Check sheet for the modelled part. Datum: model origin and axes. Units: mm. A direction names the side the tool comes from. Round coordinates to 2 decimals unless told otherwise and drop trailing zeros. Order: outer loops, then holes, each group sorted by start corner. A loop starts at its lowest first (then second) coordinate and runs counter-clockwise, first axis right, second up.
Q1. Set-up check for faces 4 (the flat face through (-301, 51, 18)), 5 (the cylindrical face through (-154, 53, 42)), 6 (the flat face through (-301, 51, -1)), 7 (the flat face through (-1, 51, 18)): record each of +Z, -Z, +X, -X, +Y, -Y from which the full face is reachable in a straight line by a thin tool's end or side.
Q2. Scan lines: probe 1 along Z at (x, y) = (-7, 50); probe 2 along Z at (x, y) = (-63.5, 12); probe 3 along X at (y, z) = (46, -14). Record each from-to range of solid material in increasing order.
Q3. Mould release check, pull along X, two halves, no side actions. Record for faces 1 (the flat face through (-152, 51, 0)), 2 (the flat face through (1, 50, -3)), 3 (the flat face through (-1, 40, -3)): +X half, -X half, draft (parallel to the pull), parting line (faces both ways), or undercut.
Q4. Depth check by flat-ended pin: P1, Ø7.5, axis at x = -261.47, y = 50, coming from the +Z side; P2, Ø5.5, axis at x = -38.53, y = 50, coming from the +Z side; P3, Ø8.5, axis at x = 38.53, y = 50, coming from the -Z side; P4, Ø4, axis at x = -305, y = 12.5, coming from the -Z side. Enter the tip coordinate at first touch or a pass-through.
Q5. Cross-section at C-C on y = 63.5. Record the cut outline in (x, z), then the cut area to 3 significant figures.
Q6. Cross-section at B-B on x = -150. Record the cut outline in (y, z).
Q7. Cross-section at A-A on z = -15. Record the cut outline in (x, y) (3 decimals).
Q8. Cross-section at D-D on z = 60. Record the cut outline in (x, y).
from build123d import *

# Parameters (mm, degrees)
SKETCH_1_R                         = 50
EXTRUDE_18_DEPTH                   = 13
EXTRUDE_18_2_DEPTH                 = 13
SKETCH_1_28_W                      = 300
SKETCH_1_28_H                      = 100
EXTRUDE_21_DEPTH                   = 15
SKETCH_1_30_R                      = 5
EXTRUDE_22_DEPTH                   = 70
SKETCH_1_31_R                      = 50
CUT_EXTRUDE_2_DEPTH                = 41
SKETCH_1_32_R                      = 50
EXTRUDE_23_DEPTH                   = 18
EXTRUDE_23_DEPTH_BACK              = 1
SKETCH_1_35_R                      = 3.175
CUT_EXTRUDE_5_DEPTH                = 130
CUT_EXTRUDE_5_DEPTH_BACK           = 69
SKETCH_1_36_R                      = 50
CUT_EXTRUDE_6_DEPTH                = 34
SKETCH_1_37_R                      = 50
EXTRUDE_24_DEPTH                   = 18
EXTRUDE_24_DEPTH_BACK              = 3
SKETCH_1_41_R                      = 3.175
CUT_EXTRUDE_7_DEPTH                = 87
CUT_EXTRUDE_7_DEPTH_BACK           = 98
THE_EXTENDED_SHAFT_CONNECTER_DEPTH = 36
SKETCH_3_R                         = 1.0922
CUT_EXTRUDE_8_DEPTH                = 31
SKETCH_5_R                         = 1.0922
SCREW_HOLES2_DEPTH                 = 47.995932


with BuildPart() as part:
    # Sketch 1 → Extrude 18 (new body)
    with BuildSketch(Plane.XY):
        with Locations((0, 50)):
            Circle(SKETCH_1_R)
    extrude(amount=EXTRUDE_18_DEPTH)



with BuildPart() as body_2:
    # Sketch 1 → Extrude 18 2 (new body)
    with BuildSketch(Plane.XY):
        with Locations((-300, 50)):
            Circle(SKETCH_1_R)
    extrude(amount=EXTRUDE_18_2_DEPTH)


with BuildPart() as part_1:
    add(part.part)

    add(body_2.part)  # Extrude 21 merges body 2
    # Sketch 1_28 → Extrude 21 (add)
    with BuildSketch(Plane.XY):
        with Locations((-150, 50)):
            Rectangle(SKETCH_1_28_W, SKETCH_1_28_H)
    extrude(amount=EXTRUDE_21_DEPTH)

    # Sketch 1_30 → Extrude 22 (add)
    with BuildSketch(Plane.XY):
        with Locations((-150, 50)):
            Circle(SKETCH_1_30_R)
    extrude(amount=EXTRUDE_22_DEPTH)

    # Sketch 1_31 → Cut-Extrude 2 (cut)
    with BuildSketch(Plane.XY):
        with Locations((-300, 50)):
            Circle(SKETCH_1_31_R)
    extrude(amount=CUT_EXTRUDE_2_DEPTH, mode=Mode.SUBTRACT)

    # Sketch 1_32 → Extrude 23 (add, two sides)
    with BuildSketch(Plane.XY) as extrude_23_sk:
        with Locations((-300, 50)):
            Circle(SKETCH_1_32_R)
    extrude(amount=EXTRUDE_23_DEPTH)
    extrude(extrude_23_sk.sketch, amount=-EXTRUDE_23_DEPTH_BACK)

    # Sketch 1_35 → Cut-Extrude 5 (cut, two sides)
    with BuildSketch(Plane.XY) as cut_extrude_5_sk:
        with Locations((-261.469660941, 50)):
            Circle(SKETCH_1_35_R)
    extrude(amount=CUT_EXTRUDE_5_DEPTH, mode=Mode.SUBTRACT)
    extrude(cut_extrude_5_sk.sketch, amount=-CUT_EXTRUDE_5_DEPTH_BACK, mode=Mode.SUBTRACT)

    # Sketch 1_36 → Cut-Extrude 6 (cut)
    with BuildSketch(Plane.XY):
        with Locations((0, 50)):
            Circle(SKETCH_1_36_R)
    extrude(amount=CUT_EXTRUDE_6_DEPTH, mode=Mode.SUBTRACT)

    # Sketch 1_37 → Extrude 24 (add, two sides)
    with BuildSketch(Plane.XY) as extrude_24_sk:
        with Locations((0, 50)):
            Circle(SKETCH_1_37_R)
    extrude(amount=EXTRUDE_24_DEPTH)
    extrude(extrude_24_sk.sketch, amount=-EXTRUDE_24_DEPTH_BACK)

    # Sketch 1_41 → Cut-Extrude 7 (cut, two sides)
    with BuildSketch(Plane.XY) as cut_extrude_7_sk:
        with Locations((-272.75493597, 77.24506403)):
            Circle(SKETCH_1_41_R)
        with BuildLine():
            ThreePointArc((-296.825, 88.530339059), (-297.75493597, 90.77540309), (-300, 91.705339059))
            Line((-300, 91.705339059), (-300, 85.355339059))
            ThreePointArc((-300, 85.355339059), (-297.75493597, 86.285275029), (-296.825, 88.530339059))
        make_face()
        with BuildLine():
            Line((-300, 85.355339059), (-300, 91.705339059))
            ThreePointArc((-300, 91.705339059), (-303.175, 88.530339059), (-300, 85.355339059))
        make_face()
        with Locations((-327.24506403, 77.24506403)):
            Circle(SKETCH_1_41_R)
        with Locations((-338.530339059, 50)):
            Circle(SKETCH_1_41_R)
        with BuildLine():
            ThreePointArc((-325, 25), (-329.490128061, 25), (-329.490128061, 20.509871939))
            Line((-329.490128061, 20.509871939), (-325, 25))
        make_face()
        with BuildLine():
            Line((-325, 25), (-329.490128061, 20.509871939))
            ThreePointArc((-329.490128061, 20.509871939), (-326.030044133, 19.821618454), (-324.07006403, 22.75493597))
            ThreePointArc((-324.07006403, 22.75493597), (-324.311746515, 23.969955867), (-325, 25))
        make_face()
        with BuildLine():
            ThreePointArc((-300, 14.644660941), (-303.175, 11.469660941), (-300, 8.294660941))
            Line((-300, 8.294660941), (-300, 14.644660941))
        make_face()
        with BuildLine():
            Line((-300, 14.644660941), (-300, 8.294660941))
            ThreePointArc((-300, 8.294660941), (-297.75493597, 9.22459691), (-296.825, 11.469660941))
            ThreePointArc((-296.825, 11.469660941), (-297.75493597, 13.714724971), (-300, 14.644660941))
        make_face()
        with Locations((-272.75493597, 22.75493597)):
            Circle(SKETCH_1_41_R)
        with BuildLine():
            ThreePointArc((-264.644660941, 50), (-261.469660941, 46.825), (-258.294660941, 50))
            Line((-258.294660941, 50), (-264.644660941, 50))
        make_face()
        with BuildLine():
            Line((-264.644660941, 50), (-258.294660941, 50))
            ThreePointArc((-258.294660941, 50), (-261.469660941, 53.175), (-264.644660941, 50))
        make_face()
        with Locations((-27.24506403, 22.75493597)):
            Circle(SKETCH_1_41_R)
        with Locations((-38.530339059, 50)):
            Circle(SKETCH_1_41_R)
        with Locations((-27.24506403, 77.24506403)):
            Circle(SKETCH_1_41_R)
        with BuildLine():
            ThreePointArc((3.175, 88.530339059), (2.24506403, 90.77540309), (0, 91.705339059))
            Line((0, 91.705339059), (0, 85.355339059))
            ThreePointArc((0, 85.355339059), (2.24506403, 86.285275029), (3.175, 88.530339059))
        make_face()
        with BuildLine():
            Line((0, 85.355339059), (0, 91.705339059))
            ThreePointArc((0, 91.705339059), (-3.175, 88.530339059), (0, 85.355339059))
        make_face()
        with Locations((27.24506403, 77.24506403)):
            Circle(SKETCH_1_41_R)
        with Locations((27.24506403, 22.75493597)):
            Circle(SKETCH_1_41_R)
        with Locations((38.530339059, 50)):
            Circle(SKETCH_1_41_R)
        with BuildLine():
            ThreePointArc((0, 14.644660941), (-3.175, 11.469660941), (0, 8.294660941))
            Line((0, 8.294660941), (0, 14.644660941))
        make_face()
        with BuildLine():
            Line((0, 14.644660941), (0, 8.294660941))
            ThreePointArc((0, 8.294660941), (2.24506403, 9.22459691), (3.175, 11.469660941))
            ThreePointArc((3.175, 11.469660941), (2.24506403, 13.714724971), (0, 14.644660941))
        make_face()
    extrude(amount=CUT_EXTRUDE_7_DEPTH, mode=Mode.SUBTRACT)
    extrude(cut_extrude_7_sk.sketch, amount=-CUT_EXTRUDE_7_DEPTH_BACK, mode=Mode.SUBTRACT)

    # Sketch 1_43 → the extended shaft connecter (add)
    with BuildSketch(Plane.XY):
        with BuildLine():
            Line((0, 43.75), (0, 40.475))
            ThreePointArc((0, 40.475), (6.735192091, 43.264807909), (9.525, 50))
            ThreePointArc((9.525, 50), (6.735192091, 56.735192091), (0, 59.525))
            Line((0, 59.525), (0, 56.25))
            ThreePointArc((0, 56.25), (3.642600233, 55.078775791), (5.919983963, 52.004068333))
            Line((5.919983963, 52.004068333), (6.25, 52.004068333))
            Line((6.25, 52.004068333), (8.25, 52.004068333))
            Line((8.25, 52.004068333), (8.25, 50))
            Line((8.25, 50), (8.25, 47.995931667))
            Line((8.25, 47.995931667), (6.25, 47.995931667))
            Line((6.25, 47.995931667), (5.919983963, 47.995931667))
            ThreePointArc((5.919983963, 47.995931667), (3.642600233, 44.921224209), (0, 43.75))
        make_face()
        with BuildLine():
            ThreePointArc((0, 59.525), (-9.525, 50), (0, 40.475))
            Line((0, 40.475), (0, 43.75))
            ThreePointArc((0, 43.75), (-6.25, 50), (0, 56.25))
            Line((0, 56.25), (0, 59.525))
        make_face()
    extrude(amount=-THE_EXTENDED_SHAFT_CONNECTER_DEPTH)

    # Sketch 3 → Cut-Extrude 8 (cut)
    with BuildSketch(Plane(origin=(0, 0, 0), x_dir=(0, 0, -1), z_dir=(1, 0, 0))):
        with Locations((32, 50)):
            Circle(SKETCH_3_R)
        with Locations((27, 50)):
            Circle(SKETCH_3_R)
    extrude(amount=-CUT_EXTRUDE_8_DEPTH, mode=Mode.SUBTRACT)

    # Sketch 5 → screw_holes2 (cut)
    with BuildSketch(Plane(origin=(0, 0, 0), x_dir=(1, 0, 0), z_dir=(0, 1, 0))):
        with Locations((0, 32)):
            Circle(SKETCH_5_R)
        with Locations((0, 27)):
            Circle(SKETCH_5_R)
    extrude(amount=SCREW_HOLES2_DEPTH, mode=Mode.SUBTRACT)


solid = part_1.part
Results found:
1. face 4: +Z, -X, +Y, -Y
1. face 5: +Z
1. face 6: -Z, -X, +Y, -Y
1. face 7: +Z, +X, +Y, -Y
2. probe 1: z = -36 to -33.09, -30.91 to -28.09, -25.91 to 18
2. probe 2: z = 0 to 15
2. probe 3: x = -8.64 to -4.8, 4.8 to 8.64
3. face 1: undercut
3. face 2: undercut
3. face 3: draft
4. P1: stops at z = 18
4. P2: passes through
4. P3: stops at z = -3
4. P4: stops at z = -1
5. outline: (-348.14, -1) - (-251.86, -1) - (-251.86, 0) - (-48.14, 0) - (-48.14, -3) - (48.14, -3) - (48.14, 18) - (-48.14, 18) - (-48.14, 15) - (-251.86, 15) - (-251.86, 18) - (-348.14, 18) - close
5. area: 6,910 mm2
6. outline: (0, 0) - (100, 0) - (100, 15) - (55, 15) - (55, 70) - (45, 70) - (45, 15) - (0, 15) - close
7. outline: circle Ø19.05 at (0, 50); hole (5.92, 47.996) - (8.25, 47.996) - (8.25, 52.004) - (5.92, 52.004) arc R6.25 ccw (long way) to start
8. outline: circle Ø10 at (-150, 50)
